Can you work these out from the model? Positions are in its coordinate system, mm. A direction names the side the tool comes from. Give positions to 0.01 mm unless a question says otherwise; leave off trailing zeros. Write each loop counter-clockwise with the first axis right and the second up, starting at its lowest first coordinate (ties: lowest second). Pieces come first, ordered by that corner, then holes.
1. I'm going to push flat-ended pins straight in: pin 1 (9.5 mm diameter, centred on x = 73.5, y = 0, fed in from +Z); pin 2 (8 mm diameter, centred on y = -15, z = 1.5, fed in from +X). Where does each tip first touch, or does it pass through?
2. On a 3-axis mill with a long thin cutter (end or side, diameter ignored), from which of +Z, -Z, +X, -X, +Y, -Y can I reach the whole of each face in a straight line? I mean faces 1 (the flat face through (45, 0, 50)), 2 (the flat face through (7, -35, 0)). Say none if no direction works.
3. Suppose I cut it at C-C (x = 73.5). Please give me the cut outline in (y, z).
4. Suppose I cut it at A-A (x = 16). Please give me the cut outline in (y, z).
5. Suppose I cut it at B-B (y = 0). Please give me the cut outline in (x, z).
6. Suppose I cut it at D-D (y = 7.5). Please give me the cut outline in (x, z).
7. If I drill on probe 1 along Z at (x, y) = (50, -11.5); probe 2 along X at (y, z) = (0, -52); probe 3 along X at (y, z) = (-11, 0.5), over which ranges is the centre line in solid material (lowest first)?
8. Thinking about a two-plate mould opening in Y: for faces 3 (the flat face through (40, 0, -60)), 4 (the cylindrical face through (79.494, 0.264, -54.93)), 5 (the flat face through (7, 35, 0)), which applies, pulls with the +Y half, pulls with the -Y half, needs draft (parallel to the pull), parting line crosses it, or undercut?
```python
from build123d import *

# Parameters (mm, degrees)
SKETCH1_W               = 70
SKETCH1_H               = 120
BOSS_EXTRUDE3_DEPTH     = 10
SKETCH3_W               = 70
SKETCH3_H               = 10
BOSS_EXTRUDE4_DEPTH     = 72
CUT_EXTRUDE1_DEPTH      = 150.49581934
CUT_EXTRUDE1_DEPTH_BACK = 150.49581934
SKETCH4_R               = 6


with BuildPart() as part:
    # Sketch1 → Boss-Extrude3 (new body)
    with BuildSketch(Plane.YZ):
        Rectangle(SKETCH1_W, SKETCH1_H)
    extrude(amount=BOSS_EXTRUDE3_DEPTH)

    # Sketch3 → Boss-Extrude4 (add)
    with BuildSketch(Plane.YZ.offset(10)):
        with Locations((0, 55)):
            Rectangle(SKETCH3_W, SKETCH3_H)
        with Locations((0, -55)):
            Rectangle(SKETCH3_W, SKETCH3_H)
    extrude(amount=BOSS_EXTRUDE4_DEPTH)

    # Sketch4 → Cut-Extrude1 (cut, two sides: drawn at the far end of the back side and taken through both)
    with BuildSketch(Plane(origin=(0, 0, -60), x_dir=(1, 0, 0), z_dir=(0, 0, -1)).offset(-CUT_EXTRUDE1_DEPTH_BACK)):
        with Locations(Location((73.5, 0, 0), (0, 0, 180))):
            Circle(SKETCH4_R)
    extrude(amount=CUT_EXTRUDE1_DEPTH + CUT_EXTRUDE1_DEPTH_BACK, mode=Mode.SUBTRACT)


solid = part.part
```
Checks:
1. pin 1: passes through
1. pin 2: stops at x = 10
2. face 1: +X, +Y, -Y
2. face 2: +Z, -Z, +X, -X, -Y
3. outline: (-35, -60) - (-6, -60) - (-6, -50) - (-35, -50) - close; (-35, 50) - (-6, 50) - (-6, 60) - (-35, 60) - close; (6, -60) - (35, -60) - (35, -50) - (6, -50) - close; (6, 50) - (35, 50) - (35, 60) - (6, 60) - close
4. outline: (-35, -60) - (35, -60) - (35, -50) - (-35, -50) - close; (-35, 50) - (35, 50) - (35, 60) - (-35, 60) - close
5. outline: (0, -60) - (67.5, -60) - (67.5, -50) - (10, -50) - (10, 50) - (67.5, 50) - (67.5, 60) - (0, 60) - close; (79.5, -60) - (82, -60) - (82, -50) - (79.5, -50) - close; (79.5, 50) - (82, 50) - (82, 60) - (79.5, 60) - close
6. outline: (0, -60) - (82, -60) - (82, -50) - (10, -50) - (10, 50) - (82, 50) - (82, 60) - (0, 60) - close
7. probe 1: z = -60 to -50, 50 to 60
7. probe 2: x = 0 to 67.5, 79.5 to 82
7. probe 3: x = 0 to 10
8. face 3: needs draft
8. face 4: undercut
8. face 5: pulls with the +Y half
